Read the model definition and answer for the solid it produces. Units are mm, in the model's axes. A direction names the side the tool comes from. Give positions to 0.01 mm unless a question says otherwise; leave off trailing zeros. Loops run counter-clockwise (first coordinate to the right, second up) from the corner with the lowest first, then second, coordinate; pieces in that order, holes last. Notation, with made-up numbers: (-25.5, 71.25) - (19.5, 71.25) arc R4 ccw to (19.5, 76.25) - close; hole circle Ø9 at (38, 74). An arc over 180 degrees is marked (long way). Write item = value, one per line.
```python
from build123d import *

# Parameters (mm, degrees)
F1_DEPTH = 4.064
F0_W     = 101.6
F0_H     = 10.16
F2_DEPTH = 20.32


with BuildPart() as f1:
    # F0 (on Front) → F1 (new body, symmetric)
    with BuildSketch(Plane.XZ):
        with BuildLine():
            ThreePointArc((153.4528778619, 203.2), (52.8306922848, 128.7287842706), (0, 15.24))
            Line((0, 15.24), (0, 10.16))
            Line((0, 10.16), (101.6, 10.16))
            Line((101.6, 10.16), (101.6, 15.24))
            Line((101.6, 15.24), (204.2528778619, 193.04))
            Line((204.2528778619, 193.04), (204.2528778619, 203.2))
            Line((204.2528778619, 203.2), (153.4528778619, 203.2))
        make_face()
        with BuildLine():
            Line((92.8011818976, 25.4), (21.2264241823, 25.4))
            ThreePointArc((21.2264241823, 25.4), (17.1886545886, 27.397336102), (16.3259964047, 31.8187335794))
            ThreePointArc((16.3259964047, 31.8187335794), (28.3591193477, 65.7147748231), (45.2871385288, 97.4508714067))
            ThreePointArc((45.2871385288, 97.4508714067), (48.3974495661, 99.6739601652), (52.177042611, 99.098777766))
            Line((52.177042611, 99.098777766), (111.9565313489, 63.5238037174))
            ThreePointArc((111.9565313489, 63.5238037174), (114.2741096305, 60.4406934976), (113.7580367399, 56.6183373538))
            Line((113.7580367399, 56.6183373538), (97.2005909488, 27.94))
            ThreePointArc((97.2005909488, 27.94), (95.3411818976, 26.0805909488), (92.8011818976, 25.4))
        make_face(mode=Mode.SUBTRACT)
        with BuildLine():
            Line((60.353951044, 116.8828291829), (151.7897789297, 139.7113057545))
            ThreePointArc((151.7897789297, 139.7113057545), (157.076894511, 137.8404624823), (157.4197225426, 132.2425955082))
            Line((157.4197225426, 132.2425955082), (123.9189236165, 74.217509674))
            ThreePointArc((123.9189236165, 74.217509674), (120.8018707091, 71.8420277322), (116.9216109051, 72.3920433103))
            Line((116.9216109051, 72.3920433103), (58.6091095788, 107.0940082349))
            ThreePointArc((58.6091095788, 107.0940082349), (56.2200964977, 110.4914552728), (57.1645380163, 114.5359651436))
            ThreePointArc((57.1645380163, 114.5359651436), (57.3571583281, 114.7887213361), (57.5501106483, 115.0412241669))
            ThreePointArc((57.5501106483, 115.0412241669), (58.795633634, 116.2001411551), (60.353951044, 116.8828291829))
        make_face(mode=Mode.SUBTRACT)
        with BuildLine():
            Line((142.5279448136, 184.912), (187.828417404, 184.912))
            Line((187.828417404, 184.912), (170.1352936925, 154.2666107871))
            ThreePointArc((170.1352936925, 154.2666107871), (168.7937516154, 152.7500297675), (166.966419203, 151.8779005407))
            Line((166.966419203, 151.8779005407), (84.0438107409, 131.1748909185))
            ThreePointArc((84.0438107409, 131.1748909185), (78.387658406, 133.6095467697), (79.2344546676, 139.7089356276))
            ThreePointArc((79.2344546676, 139.7089356276), (109.0518420167, 164.8719409502), (142.5279448136, 184.912))
        make_face(mode=Mode.SUBTRACT)
    extrude(amount=F1_DEPTH, both=True)

    # F0 (on Front) → F2 (join, symmetric)
    with BuildSketch(Plane.XZ):
        with Locations((50.8, 5.08)):
            Rectangle(F0_W, F0_H)
    extrude(amount=F2_DEPTH, both=True)


solid = f1.part
```
1) Find the intervals of material crossed by probe 1 along Z at (x, y) = (62, 16); probe 2 along Z at (x, y) = (119, -1); probe 3 along X at (y, z) = (-3.5, 90.5), in increasing order.
Output:
probe_1 = 0 to 10.16
probe_2 = 45.38 to 71.7, 131.52 to 139.9, 171.61 to 185.96
probe_3 = 27.03 to 41.05, 66.63 to 86.49, 133.32 to 145.05
2) A cutting plane is placed at B-B on y = 1.5. Give the number of separate pieces and of enclosed holes in the cut face, then the cut area to 3 significant figures.
Output:
separate_pieces = 1
enclosed_holes = 3
area = 10,000 mm²
3) The mould has two halves that part along Z. Classify faces 4 (the face through (50, 0, 0)), 5 (the face through (204.253, 0, 198)), 6 (the face through (17.229, -0.057, 27.346)): pulls with the +Z half, pulls with the -Z half, needs draft (parallel to the pull), parting line crosses it, or undercut.
Output:
face_4 = pulls with the -Z half
face_5 = needs draft
face_6 = undercut
4) A cutting plane is placed at C-C on x = 89. Determine the outline of the cut face in (y, z).
Output:
outline = (-20.32, 0) - (20.32, 0) - (20.32, 10.16) - (4.06, 10.16) - (4.06, 25.4) - (-4.06, 25.4) - (-4.06, 10.16) - (-20.32, 10.16) - close; (-4.06, 77.19) - (4.06, 77.19) - (4.06, 89.01) - (-4.06, 89.01) - close; (-4.06, 124.03) - (4.06, 124.03) - (4.06, 132.41) - (-4.06, 132.41) - close; (-4.06, 148.88) - (4.06, 148.88) - (4.06, 164.89) - (-4.06, 164.89) - close
5) A cutting plane is placed at D-D on z = 86. Determine the outline of the cut face in (x, y), then the cut area to 3 significant figures.
Output:
outline = (24.61, -4.06) - (38.47, -4.06) - (38.47, 4.06) - (24.61, 4.06) - close; (74.19, -4.06) - (94.06, -4.06) - (94.06, 4.06) - (74.19, 4.06) - close; (130.72, -4.06) - (142.45, -4.06) - (142.45, 4.06) - (130.72, 4.06) - close
area = 370 mm²
6) A cutting plane is placed at A-A on z = 142.5. Determine the outline of the cut face in (x, y), then the cut area to 3 significant figures.
Output:
outline = (64.93, -4.06) - (82.09, -4.06) - (82.09, 4.06) - (64.93, 4.06) - close; (129.4, -4.06) - (175.07, -4.06) - (175.07, 4.06) - (129.4, 4.06) - close
area = 511 mm²
7) Each of these flat-tipped pins is pushed along its axis until it touches: P1, Ø17, axis at y = 3, z = 8, coming from the +X side; P2, Ø18, axis at x = 41, y = 15.5, coming from the +Z side; P3, Ø1.5, axis at y = -2, z = 117.5, coming from the -X side; P4, Ø12, axis at x = 32.5, z = 48.5, coming from the +Y side. Where does it stop, or does it pass through?
Output:
P1 = 102.33
P2 = 10.16
P3 = 43.63
P4 = through
8) A tool of negligible diameter and unlimited length cuts with its end or side. For faces 1 (the face through (101.6, 0, 6)), 2 (the face through (165, 0, 184.912)), 3 (the face through (94.1, 4.064, 85.7)), from which of +Z, -Z, +X, -X, +Y, -Y can it reach the whole face along a straight path? Write none if from no direction.
Output:
face_1 = -Z, +X, +Y, -Y
face_2 = +Y, -Y
face_3 = +Z, +X, -X, +Y
